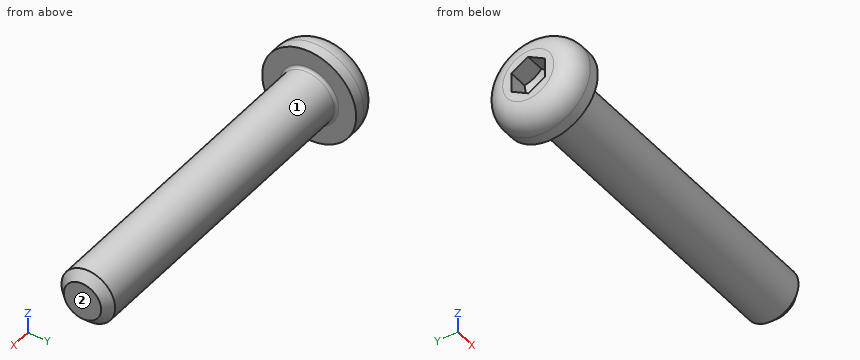
Autodesk Inventor part; units mm, degrees
ref_plane "Work Plane1" through (29, 0, 0) normal (0, -1, 0) x (1, 0, 0)
ref_plane "YZ Plane" through (0, 0, 0) normal (1, 0, 0) x (0, 1, 0)
ref_plane "XZ Plane" through (0, 0, 0) normal (0, 1, 0) x (-1, 0, 0)
sketch "Sketch1" plane through (0, 0, 0) normal (0, 0, 1) x (1, 0, 0)
  line L0 (-0.0833, 0) -> (12, 0)
  line L1 (12, 0) -> (12, 1)
  line L2 (12, 1) -> (9, 1)
  line L3 (9, 1) -> (8.6932, 1)
  line L4 (8.6932, 1) -> (0, 1)
  line L5 (0, 1) -> (0, 1.75)
  line L6 (0, 1.75) -> (-1.2, 1.75)
  line L7 (-1.2, 1.75) -> (-1.2, 0.7217)
  line L8 (-1.2, 0.7217) -> (-0.5, 0.7217)
  line L9 (-0.5, 0.7217) -> (-0.0833, 0)
  line L10 (-3.84, 0) -> (14.64, 0)
  line L11 (0, -0.35) -> (0, 2.1)
  line L12 (9, 1) -> (0, 1) construction
  dimension "d1" = 3
  dimension "d2" = 0.3068
  dimension "d3" = 1.2
  dimension "d4" = 0.7
  dimension "d5" = 60
  dimension "d6" = 2
  dimension "d7" = 2
  dimension "d8" = 1.4434
  dimension "d9" = 3.5
  dimension "d26" = 12
revolve "Body" add sketch "Sketch1" angle 360 about axis through (-0.0833, 0, 0) along (1, 0, 0)
sketch "Sketch2" plane through (-1.2, 0, 0) normal (-1, 0, 0) x (0, 0, 1)
  circle A0 centre (0, 0) radius 0.7217
  line L0 (0, -2.45) -> (0, 2.45)
  line L1 (-2.45, 0) -> (2.45, 0)
  line L2 (0.7217, 0) -> (0.3608, -0.625)
  line L3 (0.3608, -0.625) -> (-0.3608, -0.625)
  line L4 (-0.3608, -0.625) -> (-0.7217, 0)
  line L5 (-0.7217, 0) -> (-0.3608, 0.625)
  line L6 (-0.3608, 0.625) -> (0.3608, 0.625)
  line L7 (0.3608, 0.625) -> (0.7217, 0)
extrude "Slot" add sketch "Sketch2" against normal up to next contours L7 A0 | A0 L2 | L6 L0 A0 | A0 L0 L3 | L0 L6 A0 | A0 L3 L0 | L4 A0 | A0 L5
fillet "Fillet1" radius 0.8 1 edges at (-1.2, -1.75, 0)
chamfer "Chamfer1" distance 0.3067 distance2 0.3067 1 edges at (12, -1, 0) measured on face at (12, -0.02, -0.3842)
ref_plane "Work Plane1" through (29, 0, 0) normal (0, -1, 0) x (1, 0, 0)
fillet "Fillet2" radius 0.1 1 edges at (0, -1, 0)
thread "Thread2"
equation "\"d15\" = -0.5 * SPD + 0.5 * GD"
equation "\"d16\" = GUL"
equation "\"GD\" = NND"
equation "\"NLG\" = 6"
equation "\"GEL\" = 4.5"
equation "\"KOD\" = 5.7"
equation "\"KOH\" = 1.65"
equation "\"INTI\" = 1.04"
equation "\"GAL\" = 0.61345 * PTC"
equation "\"GUL\" = 0.61345 * PTC"
equation "\"BDM\" = NND"
equation "\"SW\" = 2"
equation "\"RR\" = 1.45"
equation "\"SPD\" = NND - 1.2269 * PTC"
equation "\"R\" = 0.3"
equation "\"TOA\" = 30deg"
equation "\"GD1\" = THREADDIA - 1.2269 * PTC"
equation "\"THREADDIA\" = 3"
equation "\"PTC\" = 0.5"
equation "\"NND\" = 3"
equation "\"KOH1\" = 0.2"
equation "\"E0\" = 2.303"
properties part number "M2x10 Bolt" material "Stainless Steel"
The listing builds one solid part. Answer for the finished solid, in the listing's coordinates (mm). Face numbers are marked on the shaded views. A direction names the side the tool comes from. Coordinates: 2 decimals unless noted, no trailing zeros. Write each loop counter-clockwise with the first axis right and the second up, starting at its lowest first coordinate (ties: lowest second). Pieces come first, ordered by that corner, then holes. Notation, with made-up numbers: M -10.75,50 L 31.25,50 A19 ccw 31.25,79 Z; hole C -1,0.5 d2. An arc over 180 degrees is marked long. Write each question's results on one line, items separated by ' | '.
Item 1: Given P1, Ø1, axis at x = 5, y = 1, coming from the -Z side, flat-ended and moving along its own axis, determine where the tip first touches the part or whether it passes through.
Answer below:
P1: z = -0.87
Item 2: Consider probe 1 along X at (y, z) = (-0.15, 0.45); probe 2 along Z at (x, y) = (4.75, 0.75); probe 3 along Z at (x, y) = (4.5, -0.5). Determine where each line is inside the solid, lowest interval first. Write a range as [from, to].
Answer below:
probe 1: [-0.36, 12] | probe 2: [-0.66, 0.66] | probe 3: [-0.87, 0.87]
Item 3: The part is cut by section A-A on x = 10.5. Determine the outline of the cut face in (y, z), and give its area (3 significant figures).
Answer below:
outline: C 0,0 d2 | area: 3.14 mm2
Item 4: Which of the six approach directions +Z, -Z, +X, -X, +Y, -Y give full straight-line access (tool end or side, diameter ignored) to the marked faces 1 and 2?
Answer below:
face 1: +X | face 2: +Z, -Z, +X, +Y, -Y
